Build history of the part. All positions in model axes, mm. A direction names the side the tool comes from. Round coordinates to 2 decimals unless told otherwise and drop trailing zeros. Order: outer loops, then holes, each group sorted by start corner. A loop starts at its lowest first (then second) coordinate and runs counter-clockwise, first axis right, second up. Notation, with made-up numbers: M 20,-1 L 58,-1 A9 ccw 58,8 Z; hole C 69,85.5 d2. An arc over 180 degrees is marked long. One line per item, written item: value. Start each with the question number.
Item 1: Pin check, flat tip, straight feed: pin 1 (14.5 mm diameter, centred on y = 46, z = -19.5, fed in from +X). Stop position of the tip, or through.
Item 2: Tool access for faces 1 (the flat face through (26, 44, 16.833)), 2 (the flat face through (-16.404, 54, -3)): list every direction of +Z, -Z, +X, -X, +Y, -Y with a clear straight run to the whole face (end or side of a thin tool).
Item 3: Band-saw the part on D-D, the plane y = 52. Write the cut outline in (x, z), then the cut area to 3 significant figures.
Item 4: Band-saw the part on C-C, the plane z = -6.5. Write the cut outline in (x, y).
Item 5: Band-saw the part on A-A, the plane y = 61. Write the cut outline in (x, z), then the cut area to 3 significant figures.
Item 6: Band-saw the part on B-B, the plane x = -8. Write the cut outline in (y, z), then the cut area to 3 significant figures.
Item 7: Probe L1, parallel to Z at x = -12.5, y = 68; L2, parallel to X at y = 59.5, z = 14.5. List the from-to ranges inside material, lowest first.
```python
from build123d import *

# Parameters (mm, degrees)
SKETCH1_W           = 2
SKETCH1_H           = 48
SKETCH1_H_2         = 2
SKETCH1_W_2         = 88
BOSS_EXTRUDE1_DEPTH = 90
CUT_EXTRUDE1_REACH  = 133.53


with BuildPart() as part:
    # Sketch1 → Boss-Extrude1 (new body)
    with BuildSketch(Plane(origin=(0, 0, 0), x_dir=(1, 0, 0), z_dir=(0, 1, 0))):
        with Locations((-17.403694266, 9.167350329)):
            Rectangle(SKETCH1_W, SKETCH1_H)
        with Locations((-17.403694266, -15.832649671)):
            Rectangle(SKETCH1_W, SKETCH1_H_2)
        with Locations((27.596305734, -15.832649671)):
            Rectangle(SKETCH1_W_2, SKETCH1_H_2)
    extrude(amount=BOSS_EXTRUDE1_DEPTH)

    # Sketch2 → Cut-Extrude1 (cut, up to next)
    with BuildSketch(Plane.ZY.offset(18.403694266), mode=Mode.PRIVATE) as cut_extrude1_sk1:
        Polygon((-33.167350329, 90), (5.03538313, 0), (-33.167350329, 0), align=None)
    cut_extrude1_tool1 = extrude(cut_extrude1_sk1.sketch, amount=-CUT_EXTRUDE1_REACH, mode=Mode.PRIVATE) & part.part
    add(cut_extrude1_tool1.solids().sort_by_distance((-18.403694, 30, -20.433106))[0], mode=Mode.SUBTRACT)


solid = part.part
```
Output:
1. pin 1: stops at x = -16.4
2. face 1: +Z, +X, -X, +Y, -Y
2. face 2: -Z, +X, +Y, -Y
3. outline: M -18.4,-17.04 L -16.4,-17.04 L -16.4,14.83 L 71.6,14.83 L 71.6,16.83 L -18.4,16.83 Z
3. area: 244 mm²
4. outline: M -18.4,27.18 L -16.4,27.18 L -16.4,90 L -18.4,90 Z
5. outline: M -18.4,-20.86 L -16.4,-20.86 L -16.4,14.83 L 71.6,14.83 L 71.6,16.83 L -18.4,16.83 Z
5. area: 251 mm²
6. outline: M 0,14.83 L 90,14.83 L 90,16.83 L 0,16.83 Z
6. area: 180 mm²
7. L1: z = 14.83 to 16.83
7. L2: x = -18.4 to -16.4
